Verification items for this drawing (mm, ordinates from the low corner). Give positions to 0.01 mm unless a question says otherwise; leave off trailing zeros. Loops run counter-clockwise (first coordinate to the right, second up) from the corner with the lowest first, then second, coordinate; pieces in that order, holes last. Notation, with made-up numbers: (-19, 64.25) - (8, 64.25) arc R24 ccw to (8, 78.25) - close; hole circle Ø3 at (-36.75, 15). An arc over 180 degrees is marked (long way). Write item = value, one per line. Start each with the question number.
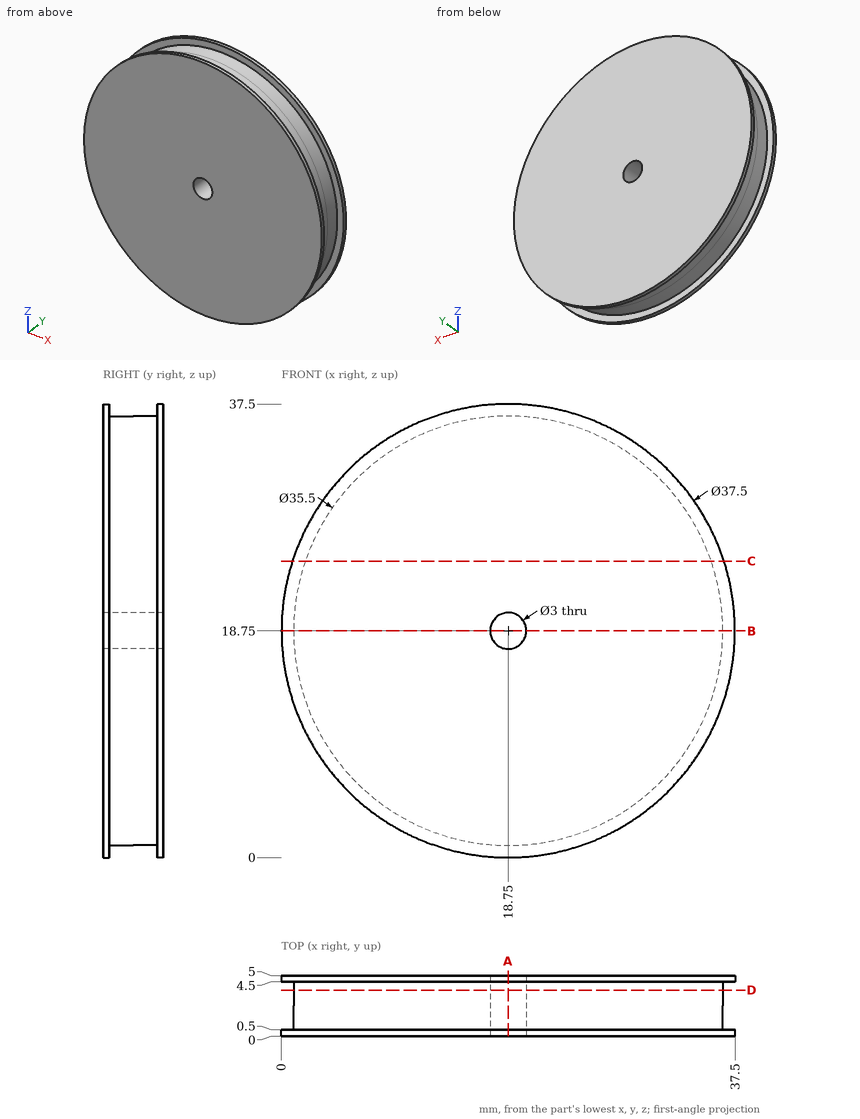
1) Cross-section at C-C on z = 24.5. Enter the section's corners in (x, y).
2) Material ranges on line 1 along Z through (x, y) = (18.75, 2.8); line 2 along Z through (x, y) = (6.5, 2.2), recorded low to high.
3) Cross-section at A-A on x = 18.75. Enter the section's corners in (y, z), and give its area (4 significant figures).
4) Cross-section at B-B on z = 18.75. Enter the section's corners in (x, y), and give its area (4 significant figures).
5) Cross-section at D-D on y = 3.8. Enter the section's corners in (x, z), and give its area (3 significant figures).
6) Gauge pin test, flat ends, axial feed: P1, Ø1.5, axis at x = 19.5, y = 2.5, coming from the +Z side; P2, Ø2, axis at y = 4.5, z = 30, coming from the +X side. Record the tip position at first contact, or that the pin passes through.
Checked values:
q1.outline = (0.9, 0) - (36.6, 0) - (36.6, 0.5) - (35.54, 0.5) - (35.54, 4.5) - (36.6, 4.5) - (36.6, 5) - (0.9, 5) - (0.9, 4.5) - (1.96, 4.5) - (1.96, 0.5) - (0.9, 0.5) - close
q2.line_1 = 1 to 17.25, 20.25 to 36.5
q2.line_2 = 5.9 to 31.6
q3.outline = (0, 0) - (0.5, 0) - (0.5, 1) - (4.5, 1) - (4.5, 0) - (5, 0) - (5, 17.25) - (0, 17.25) - close; (0, 20.25) - (5, 20.25) - (5, 37.5) - (4.5, 37.5) - (4.5, 36.5) - (0.5, 36.5) - (0.5, 37.5) - (0, 37.5) - close
q3.area = 164.5 mm²
q4.outline = (0, 0) - (17.25, 0) - (17.25, 5) - (0, 5) - (0, 4.5) - (1, 4.5) - (1, 0.5) - (0, 0.5) - close; (20.25, 0) - (37.5, 0) - (37.5, 0.5) - (36.5, 0.5) - (36.5, 4.5) - (37.5, 4.5) - (37.5, 5) - (20.25, 5) - close
q4.area = 164.5 mm²
q5.outline = circle Ø35.5 at (18.75, 18.75); hole circle Ø3 at (18.75, 18.75)
q5.area = 983 mm²
q6.P1 = 36.5
q6.P2 = 34.45
